Answer from the drawing. Dimensions are ordinates in mm from the lowest x, y and z of the part. A direction names the side the tool comes from. Round coordinates to 2 decimals unless told otherwise and drop trailing zeros. Order: outer loops, then holes, each group sorted by start corner. A loop starts at its lowest first (then second) coordinate and runs counter-clockwise, first axis right, second up. Notation, with made-up numbers: (15, 66) -> (65, 66) arc R23 cw to (65, 104) -> close; hole circle Ø9 at (-14, 53). An arc over 180 degrees is marked (long way). Use a Markdown table: item, result. Add a question column.
1. Section C-C, the plane z = 2.25 is taken. Give the number of separate pieces and of enclosed holes in the cut face, then the cut area to 3 significant figures.
2. For the marked faces 1, 2 and 3, determine the directions among +Z, -Z, +X, -X, +Y, -Y from which every point of the face is accessible in a straight line to the end or side of a thin tool.
3. Given pin 1 (2 mm diameter, centred on y = 6.5, z = 2.5, fed in from -X); pin 2 (5 mm diameter, centred on x = 22.4, y = 18.7, fed in from +Z), each flat-ended and moving along its own axis, determine where each tip first touches the part or whether it passes through.
4. Section A-A, the plane x = 60 is taken. Give the vertices of the cut face in (y, z).
5. Consider L1, parallel to Y at x = 22.4, z = 3.9; L2, parallel to Y at x = 1.45, z = 3.5; L3, parallel to Z at x = 2, y = 30. Determine where each line is inside the solid, lowest interval first. Write a range as [from, to].
6. Section B-B, the plane y = 45.5 is taken. Give the vertices of the cut face in (x, z), then the cut area to 3 significant figures.
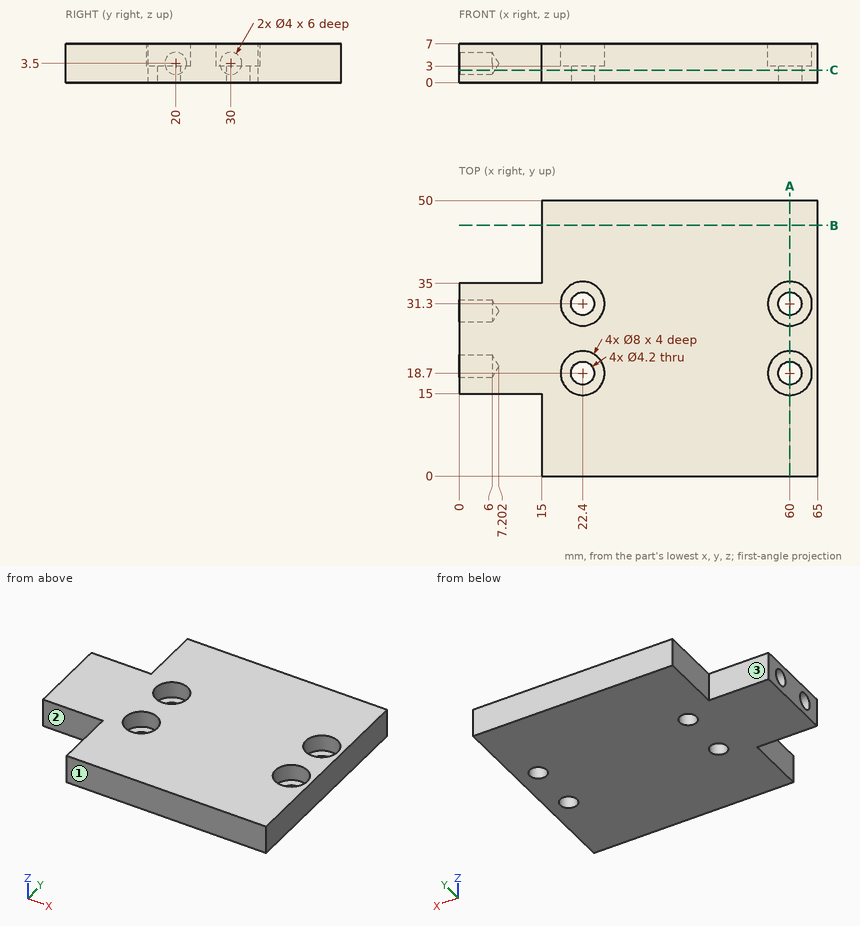
Verdict:
| question | item | result |
|---|---|---|
| 1 | separate pieces | 1 |
| 1 | enclosed holes | 4 |
| 1 | area | 2,710 mm2 |
| 2 | face 1 | +Z, -Z, +X, -X, -Y |
| 2 | face 2 | +Z, -Z, -X, -Y |
| 2 | face 3 | +Z, -Z, -X, +Y |
| 3 | pin 1 | stops at x = 15 |
| 3 | pin 2 | stops at z = 3 |
| 4 | outline | (0, 0) -> (16.6, 0) -> (16.6, 3) -> (14.7, 3) -> (14.7, 7) -> (0, 7) -> close; (20.8, 0) -> (29.2, 0) -> (29.2, 3) -> (27.3, 3) -> (27.3, 7) -> (22.7, 7) -> (22.7, 3) -> (20.8, 3) -> close; (33.4, 0) -> (50, 0) -> (50, 7) -> (35.3, 7) -> (35.3, 3) -> (33.4, 3) -> close |
| 5 | L1 | y = [0, 14.7], [22.7, 27.3], [35.3, 50] |
| 5 | L2 | y = [15, 18], [22, 28], [32, 35] |
| 5 | L3 | z = [0, 1.5], [5.5, 7] |
| 6 | outline | (15, 0) -> (65, 0) -> (65, 7) -> (15, 7) -> close |
| 6 | area | 350 mm2 |
